Autodesk Inventor part; units mm, degrees
ref_plane "YZ Plane" through (0, 0, 0) normal (1, 0, 0) x (0, 1, 0)
ref_plane "XZ Plane" through (0, 0, 0) normal (0, 1, 0) x (-1, 0, 0)
ref_plane "XY Plane" through (0, 0, 0) normal (0, 0, 1) x (1, 0, 0)
sketch "Sketch1" plane through (0, 0, 0) normal (0, 0, 1) x (1, 0, 0)
  circle A0 centre (0, 0) radius 14.31
  line L0 (-78.5772, -49.1858) -> (-49.3914, -20)
  line L1 (0, -92.6578) -> (0, 38.7763)
  line L2 (0, -20) -> (-53.8815, -73.8815)
  line L3 (-53.8815, -73.8815) -> (-78.5772, -49.1858)
  line L4 (0, 20) -> (-103.6841, 20)
  line L5 (-103.6841, 20) -> (-157.5656, -33.8815)
  line L6 (-157.5656, -33.8815) -> (-132.8699, -58.5772)
  line L7 (-132.8699, -58.5772) -> (-94.2927, -20)
  line L8 (-94.2927, -20) -> (-49.3914, -20)
  line L9 (78.5772, -49.1858) -> (49.3914, -20)
  line L10 (0, -20) -> (53.8815, -73.8815)
  line L11 (53.8815, -73.8815) -> (78.5772, -49.1858)
  line L12 (0, 20) -> (103.6841, 20)
  line L13 (103.6841, 20) -> (157.5656, -33.8815)
  line L14 (157.5656, -33.8815) -> (132.8699, -58.5772)
  line L15 (132.8699, -58.5772) -> (94.2927, -20)
  line L16 (94.2927, -20) -> (49.3914, -20)
  line L17 (0, -20) -> (-10.1971, -30.1971)
  point P0 (-68.6659, -39.2745)
  dimension "d1" = 28.62
  dimension "d4" = 76.2
  dimension "d6" = 45
  dimension "d15" = 34.925
  dimension "d59" = 34.925
  dimension "d61" = 101.6
  dimension "d62" = 40
  dimension "d63" = 20
extrude "Extrusion1" add sketch "Sketch1" along normal blind 3.175 contours A0 L1 L12 L13 L14 L15 L16 L9 L11 L10 | A0 L1 L2 L3 L0 L8 L7 L6 L5 L4
sketch "Sketch3" plane through (0, 0, 3.175) normal (0, 0, 1) x (1, 0, 0)
  line L0 (53.8815, -73.8815) -> (78.5772, -49.1858)
  line L1 (78.5772, -49.1858) -> (49.3914, -20)
  line L2 (49.3914, -20) -> (94.2927, -20)
  line L3 (94.2927, -20) -> (132.8699, -58.5772)
  line L4 (132.8699, -58.5772) -> (157.5656, -33.8815)
  line L5 (157.5656, -33.8815) -> (103.6841, 20)
  line L6 (103.6841, 20) -> (-103.6841, 20)
  line L7 (-103.6841, 20) -> (-157.5656, -33.8815)
  line L8 (-157.5656, -33.8815) -> (-132.8699, -58.5772)
  line L9 (-132.8699, -58.5772) -> (-94.2927, -20)
  line L10 (-94.2927, -20) -> (-49.3914, -20)
  line L11 (-49.3914, -20) -> (-78.5772, -49.1858)
  line L12 (-78.5772, -49.1858) -> (-53.8815, -73.8815)
  line L13 (-53.8815, -73.8815) -> (0, -20)
  line L14 (0, -20) -> (53.8815, -73.8815)
  circle A0 centre (0, 0) radius 14.31
  line L15 (-145.2178, -46.2294) -> (-75.3998, 20)
  line L16 (-66.2294, -61.5337) -> (19.7221, 20)
  circle A1 centre (-136.0007, -37.486) radius 2.65
  circle A2 centre (-117.5728, -20.0053) radius 2.65
  circle A3 centre (-99.1449, -2.5246) radius 2.65
  circle A4 centre (-57.0123, -52.7903) radius 2.65
  circle A5 centre (-38.5844, -35.3096) radius 2.65
  circle A6 centre (-20.1566, -17.8289) radius 2.65
  dimension "d64" = 5.3
  dimension "d67" = 25.4
  dimension "d72" = 12.7
  dimension "d73" = 12.7
  dimension "d76" = 25.4
extrude "Extrusion3" cut sketch "Sketch3" against normal blind 25.4 contours A4 L16 | L16 A4 | A5 L16 | L16 A5 | A6 L16 | L16 A6 | A3 L15 | L15 A3 | A1 L15 | L15 A1 | A2 L15 | L15 A2
mirror "Mirror2" about plane through (0, 0, 0) normal (1, 0, 0) of "Extrusion3"
equation "\"d1\" = bearingDiameter"
equation "\"d4\" = boltedLength"
equation "\"d6\" = 0.5 * theta12"
equation "\"d59\" = d15"
equation "\"d61\" = gearboxLength"
equation "\"d62\" = plateHeight"
equation "\"topDiameter\" = 45"
equation "\"bearingDiameter\" = 28.62"
equation "\"plateThickness\" = 6.35"
equation "\"theta12\" = 90deg"
equation "\"gearboxLength\" = 101.6"
equation "\"boltedLength\" = 76.2"
equation "\"topDiameter_1\" = 25"
equation "\"shaftLength_1\" = 76.2"
equation "\"bearingDiameter_1\" = 28.62"
equation "\"plateThickness_1\" = 6.35"
equation "\"theta12_1\" = 100deg"
equation "\"boltDiameter_1\" = 6"
equation "\"gearboxLength_1\" = 101.6"
equation "\"boltedLength_1\" = 76.2"
equation "\"innerBoltSpacing_1\" = 12.7"
equation "\"outerBoltSpacing_1\" = 12.7"
equation "\"shaftLength\" = 76.2"
equation "\"boltDiameter\" = 5.3"
equation "\"outerBoltSpacing\" = 12.7"
equation "\"innerBoltSpacing\" = 12.7"
equation "\"plateHeight\" = 40"
properties part number "CH1-01-KneePivotPlate" material "Aluminum 6061"
Read the model definition and answer for the solid it produces. Units are mm, in the model's axes. A direction names the side the tool comes from. Give positions to 0.01 mm unless a question says otherwise; leave off trailing zeros. Loops run counter-clockwise (first coordinate to the right, second up) from the corner with the lowest first, then second, coordinate; pieces in that order, holes last.
Item 1: The part is cut by section B-B (y = -9). Write down the section's boundary in (x, z) (3 decimals), and give its area (3 significant figures).
Item 2: Find the intervals of material crossed by line 1 along X through (y, z) = (-27.5, 2.8); line 2 along X through (y, z) = (-47.5, 2.55); line 3 along X through (y, z) = (-34, 2.1), in increasing order.
Item 3: The mould has two halves that part along Y. Classify faces 1 (the flat face through (-130.248, -6.564, 1.565)), 2 (the cylindrical face through (22.26, -16.22, 1.61)), 3 (the flat face through (-2, -16, 0)), 4 (the cylindrical face through (-101.248, -4.137, 1.61)): released by +Y, released by -Y, zero draft, split by the parting line, or undercut.
Item 4: The part is cut by section C-C (z = 0.9). Give the number of separate pieces and of enclosed holes in the cut face, and give its area (3 significant figures).
Item 5: The part is cut by section A-A (x = 5). Write down the section's boundary in (y, z) (3 decimals), and give its area (3 significant figures).
Item 6: Each of these flat-tipped pins is pushed along its axis until it touches: pin 1 Ø3 at (x, y) = (20.16, -17.83) entering from +Z; pin 2 Ø1.5 at (y, z) = (-24, 1) entering from +X; pin 3 Ø1 at (x, z) = (62, 1.5) entering from -Y. Where does it stop, or does it pass through?
Item 7: For faces 5 (the flat face through (64.19, -34.8, 1.57)), 6 (the flat face through (113.85, -39.56, 1.57)), determine the directions among +Z, -Z, +X, -X, +Y, -Y from which every point of the face is accessible in a straight line to the end or side of a thin tool.
Taken from the geometry:
1. outline: (-132.684, 0) - (-11.125, 0) - (-11.125, 3.175) - (-132.684, 3.175) - close; (11.125, 0) - (132.684, 0) - (132.684, 3.175) - (11.125, 3.175) - close
1. area: 772 mm2
2. line 1: x = -151.18 to -101.79, -56.89 to -7.5, 7.5 to 56.89, 101.79 to 151.18
2. line 2: x = -143.95 to -121.79, -76.89 to -27.5, 27.5 to 76.89, 121.79 to 143.95
2. line 3: x = -157.45 to -108.29, -63.39 to -40.89, -36.28 to -14, 14 to 36.28, 40.89 to 63.39, 108.29 to 157.45
3. face 1: released by +Y
3. face 2: undercut
3. face 3: zero draft
3. face 4: undercut
4. separate pieces: 1
4. enclosed holes: 13
4. area: 15,700 mm2
5. outline: (-25, 0) - (-13.408, 0) - (-13.408, 3.175) - (-25, 3.175) - close; (13.408, 0) - (20, 0) - (20, 3.175) - (13.408, 3.175) - close
5. area: 57.7 mm2
6. pin 1: passes through
6. pin 2: stops at x = 148.43
6. pin 3: stops at y = -66.26
7. face 5: +Z, -Z
7. face 6: +Z, -Z, -Y
